```python
from build123d import *

# Parameters (mm, degrees)
F0_R     = 207.035433
F1_DEPTH = 12
F3_D     = 85
F6_D     = 8


with BuildPart() as f1:
    # F0 (on Top) → F1 (new body)
    with BuildSketch(Plane.XY):
        Circle(F0_R)
    extrude(amount=F1_DEPTH)

    # F3 (through all)
    with Locations(Plane(origin=(0, 0, 0), x_dir=(1, 0, 0), z_dir=(0, 0, -1))):
        with Locations((0, 0)):
            Hole(F3_D / 2)

    # F6 (through all)
    with Locations(Plane(origin=(0, 0, 0), x_dir=(1, 0, 0), z_dir=(0, 0, -1))):
        with Locations((-75.952627, 0), (-39.412599, 65.299459), (42.192809, 63.676074), (76.147959, 0), (37.442353, -66.324979), (-44.154473, -61.992928)):
            Hole(F6_D / 2)


solid = f1.part
```
Can you work these out from the model? Positions are in its coordinate system, mm. Coordinates: 2 decimals unless noted, no trailing zeros. Loops run counter-clockwise (first coordinate to the right, second up) from the corner with the lowest first, then second, coordinate; pieces in that order, holes last. Notation, with made-up numbers: (-24.75, 25.5) -> (-7.75, 25.5) arc R18 cw to (-7.75, 53.5) -> close; hole circle Ø7 at (-28.75, 11.5). An arc over 180 degrees is marked (long way). Put each result on its own line as item: value. Start each with the question number.
Q1. I'm going to push flat-ended pins straight in: P1, Ø6, axis at x = -93.5, z = 6.5, coming from the +Y side; P2, Ø13, axis at x = 42.19, y = -63.68, coming from the +Z side; P3, Ø6, axis at y = -36.5, z = 3.5, coming from the +X side; P4, Ø5, axis at x = -34.5, z = 4, coming from the -Y side. Where does each tip first touch, or does it pass through?
Q2. If I drill on line 1 (Y direction, x = -2.5, z = 3.75); line 2 (Y direction, x = 25.5, z = 3.75); line 3 (X direction, y = -12.5, z = 8.25), over which ranges is the centre line in solid material (lowest first)? Write a range as [from, to].
Q3. Thinking about a two-plate mould opening in X: for faces 1 (the face through (33.727, 25.861, 6.084)), 2 (the face through (-44.881, -202.112, 5.916)), 3 (the face through (-3, -43, 12)), which applies, pulls with the +X half, pulls with the -X half, needs draft (parallel to the pull), parting line crosses it, or undercut?
Q4. I want a section at A-A (x = 0). Write out the boundary of the cut face in (y, z), plus the area to 3 significant figures.
Q5. I want a section at D-D (x = -165). Write out the boundary of the cut face in (y, z), plus the area to 3 significant figures.
Q6. I want a section at C-C (y = 117.5). Write out the boundary of the cut face in (x, z), plus the area to 3 significant figures.
Q7. I want a section at B-B (z = 5.75). Write out the boundary of the cut face in (x, y).
Taken from the geometry:
1. P1: stops at y = 186.21
1. P2: stops at z = 12
1. P3: stops at x = 204.31
1. P4: stops at y = -204.55
2. line 1: y = [-207.02, -42.43], [42.43, 207.02]
2. line 2: y = [-205.46, -34], [34, 205.46]
2. line 3: x = [-206.66, -40.62], [40.62, 206.66]
3. face 1: undercut
3. face 2: parting line crosses it
3. face 3: needs draft
4. outline: (-207.04, 0) -> (-42.5, 0) -> (-42.5, 12) -> (-207.04, 12) -> close; (42.5, 0) -> (207.04, 0) -> (207.04, 12) -> (42.5, 12) -> close
4. area: 3,950 mm2
5. outline: (-125.05, 0) -> (125.05, 0) -> (125.05, 12) -> (-125.05, 12) -> close
5. area: 3,000 mm2
6. outline: (-170.46, 0) -> (170.46, 0) -> (170.46, 12) -> (-170.46, 12) -> close
6. area: 4,090 mm2
7. outline: circle Ø414.07 at (0, 0); hole circle Ø8 at (-75.95, 0); hole circle Ø8 at (-44.15, 61.99); hole circle Ø8 at (-39.41, -65.3); hole circle Ø85 at (0, 0); hole circle Ø8 at (37.44, 66.32); hole circle Ø8 at (42.19, -63.68); hole circle Ø8 at (76.15, 0)
